from build123d import *

# Parameters (mm, degrees)
SKETCH1_W            = 150
SKETCH1_H            = 6
BOSS_EXTRUDE1_DEPTH  = 6
SKETCH1_3_W          = 38
SKETCH1_3_H          = 14.35
BOSS_EXTRUDE2_DEPTH  = 3
M3_CLEARANCE_HOLE1_D = 3.6
FILLET1_R            = 6
FILLET2_R            = 2


with BuildPart() as part:
    # Sketch1 → Boss-Extrude1 (new body)
    with BuildSketch(Plane.XY):
        with Locations((75, 3)):
            Rectangle(SKETCH1_W, SKETCH1_H)
    extrude(amount=BOSS_EXTRUDE1_DEPTH)

    # Sketch1<3> → Boss-Extrude2 (add)
    with BuildSketch(Plane.XY):
        with Locations((67.63, 13.175)):
            Rectangle(SKETCH1_3_W, SKETCH1_3_H)
    extrude(amount=BOSS_EXTRUDE2_DEPTH)

    # M3 Clearance Hole1 (through all)
    with Locations(Plane.XY.offset(3)):
        with Locations((52.63, 16.35), (82.63, 16.35)):
            Hole(M3_CLEARANCE_HOLE1_D / 2)

    # Fillet1
    fillet1_edges = [part.edges().sort_by_distance(p)[0] for p in [
        (150, 0, 3),
        (0, 0, 3),
    ]]
    fillet(fillet1_edges, radius=FILLET1_R - 0.0001)  # a hair under: the kernel refuses the full size

    # Fillet2
    fillet2_edges = [part.edges().sort_by_distance(p)[0] for p in [
        (86.63, 6, 1.5),
        (86.63, 20.35, 1.5),
        (48.63, 20.35, 1.5),
        (48.63, 6, 1.5),
        (0, 6, 3),
        (150, 6, 3),
    ]]
    fillet(fillet2_edges, radius=FILLET2_R)


solid = part.part
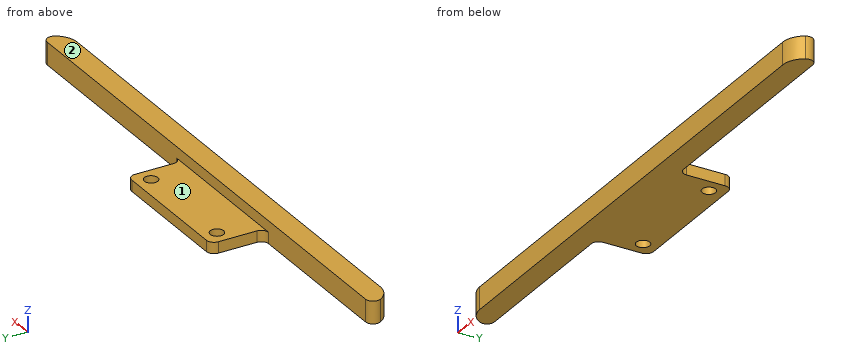
Geometry check sheet. Reference: the model listing, model coordinates, mm. Face numbers are marked on the shaded views. A direction names the side the tool comes from. Round coordinates to 2 decimals unless told otherwise and drop trailing zeros. Loops run counter-clockwise (first coordinate to the right, second up) from the corner with the lowest first, then second, coordinate; pieces in that order, holes last. Notation, with made-up numbers: (58.5, -22.75) - (102.5, -22.75) arc R17 ccw to (102.5, -15.75) - close; hole circle Ø7 at (67.5, 86.5). An arc over 180 degrees is marked (long way). One line per question, with ' | ' between items. Start each with the question number.
1. Cross-section at A-A on x = 52.63. Record the cut outline in (y, z).
2. Cross-section at C-C on x = 74.5. Record the cut outline in (y, z), then the cut area to 4 significant figures.
3. Cross-section at D-D on z = 1. State how many separate pieces and enclosed holes the cut face has, then the cut area to 3 significant figures.
4. Tool access check on the marked faces 1 and 2. Record the directions out of +Z, -Z, +X, -X, +Y, -Y that give a thin tool (end or side, any length) a straight path to the whole face; none if there is none.
5. Depth check by flat-ended pin: pin 1 (1.5 mm diameter, centred on x = 41, z = 4, fed in from +Y); pin 2 (1.5 mm diameter, centred on y = 14, z = 1, fed in from -X); pin 3 (1.5 mm diameter, centred on y = 12.5, z = 1, fed in from +X). Enter the tip coordinate at first touch or a pass-through.
6. Cross-section at B-B on y = 16.35. Record the cut outline in (x, z).
7. Scan lines: line 1 (X direction, y = 17.25, z = 2); line 2 (Y direction, x = 52.63, z = 1.2); line 3 (Y direction, x = 125, z = 1.75). Record each from-to range of solid material in increasing order. Write a range as [from, to].
Taken from the geometry:
1) outline: (0, 0) - (14.55, 0) - (14.55, 3) - (6, 3) - (6, 6) - (0, 6) - close; (18.15, 0) - (20.35, 0) - (20.35, 3) - (18.15, 3) - close
2) outline: (0, 0) - (20.35, 0) - (20.35, 3) - (6, 3) - (6, 6) - (0, 6) - close | area: 79.05 mm²
3) separate pieces: 1 | enclosed holes: 2 | area: 1,410 mm²
4) face 1: +Z, +X, -X, +Y | face 2: +Z, +X, -X, +Y, -Y
5) pin 1: y = 6 | pin 2: x = 48.63 | pin 3: x = 86.63
6) outline: (48.63, 0) - (50.83, 0) - (50.83, 3) - (48.63, 3) - close; (54.43, 0) - (80.83, 0) - (80.83, 3) - (54.43, 3) - close; (84.43, 0) - (86.63, 0) - (86.63, 3) - (84.43, 3) - close
7) line 1: [48.63, 51.07], [54.19, 81.07], [84.19, 86.63] | line 2: [0, 14.55], [18.15, 20.35] | line 3: [0, 6]
